```python
from build123d import *

# Parameters (mm, degrees)
F1_DEPTH = 5.842
F2_R     = 2.452841


with BuildPart() as f1:
    # F0 (on Front) → F1 (new body)
    with BuildSketch(Plane.XZ):
        with BuildLine():
            ThreePointArc((0, 28.678283), (6.286108, -2.530437), (0, -33.739157))
            ThreePointArc((0, -33.739157), (36.877814, -2.530437), (0, 28.678283))
        make_face()
    extrude(amount=F1_DEPTH)

    # F2
    f2_edges = [f1.edges().sort_by_distance(p)[0] for p in [
        (6.286108, -5.842, -2.530437),
        (36.877814, -5.842, -2.530437),
        (36.877814, 0, -2.530437),
        (6.286108, 0, -2.530437),
    ]]
    fillet(f2_edges, radius=F2_R)


solid = f1.part
```
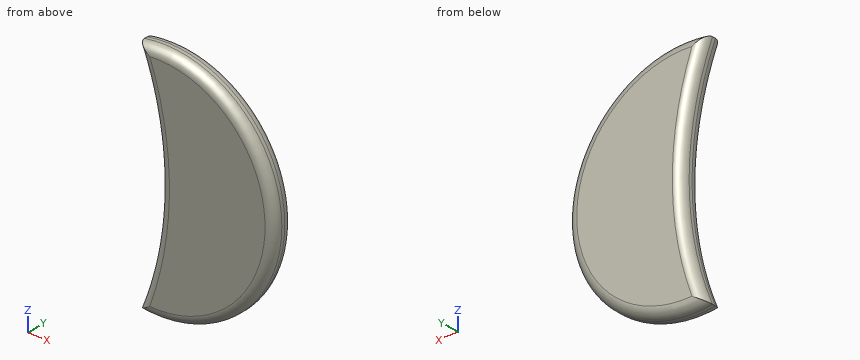
Build history of the part. All positions in model axes, mm. Give positions to 0.01 mm unless a question says otherwise; leave off trailing zeros. Order: outer loops, then holes, each group sorted by start corner. A loop starts at its lowest first (then second) coordinate and runs counter-clockwise, first axis right, second up. Notation, with made-up numbers: M 57.25,-15 L 92.25,-15 A20 cw 92.25,10 Z; hole C 30.5,84.25 d6. An arc over 180 degrees is marked long. Return JSON: item names as keys, results as strings.
Q1. Flat gauge pins, fed straight in: pin 1 (1 mm diameter, centred on x = 15, y = -0.5, fed in from +Z); pin 2 (1 mm diameter, centred on x = 23, y = -4, fed in from +Z); pin 3 (5 mm diameter, centred on x = 29, z = -24.5, fed in from +Y). Where does each tip first touch, or does it go through?
Answer list:
{"pin 1": "stops at z = 27.1", "pin 2": "stops at z = 23.92", "pin 3": "stops at y = -0.09"}
Q2. Wall check: probe 1 along X at (y, z) = (-3.35, 16); probe 2 along Z at (x, y) = (9, -5.1); probe 3 along Z at (x, y) = (10.5, -0.25). Give the ranges that are in metal, low to high. Write a range as from..to.
Answer list:
{"probe 1": "x = 4.13..30.88", "probe 2": "z = -33.25..28.19", "probe 3": "z = -32.34..27.28"}
Q3. Band-saw the part on B-B (y = -4.65). Give the cut face in (x, z), then the cut area to 3 significant figures.
Answer list:
{"outline": "M 0.49,-33.46 A31.3 ccw long 0.49,28.4 A80.96 cw Z", "area": "1,580 mm^2"}
Q4. Band-saw the part on A-A (y = -1.65). Give the cut face in (x, z), then the cut area to 3 significant figures.
Answer list:
{"outline": "M 0.19,-33.63 A31.51 ccw long 0.19,28.57 A80.75 cw Z", "area": "1,620 mm^2"}
